Drawing for the job (mm, zero at the part's lowest x, y, z). A direction names the side the tool comes from. Coordinates: 2 decimals unless noted, no trailing zeros. Order: outer loops, then holes, each group sorted by start corner. A loop starts at its lowest first (then second) coordinate and runs counter-clockwise, first axis right, second up. Notation, with made-up numbers: (-15, 14.25) - (-5, 14.25) arc R20 ccw to (-5, 52.25) - close; hole circle Ø3 at (68, 19). An arc over 180 degrees is marked (long way). Answer as CSV lines item,"result". Start each with the question number.
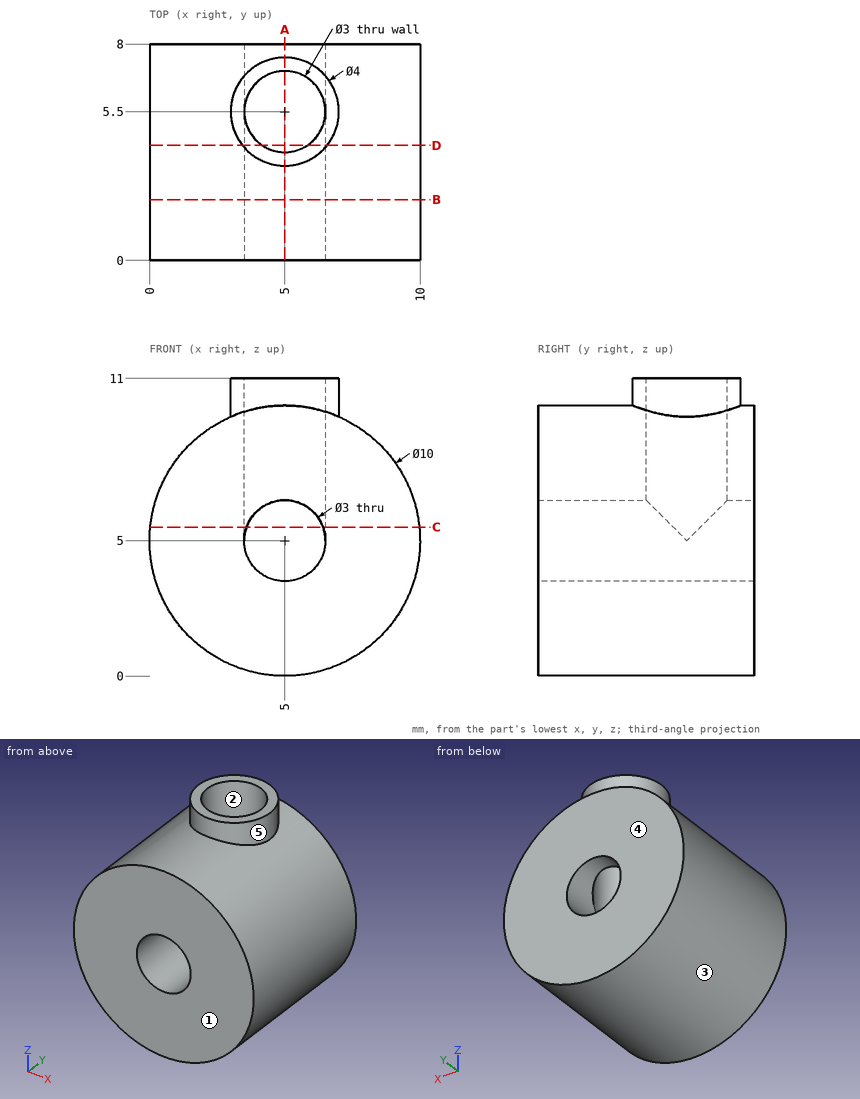
(1) Band-saw the part on D-D on y = 4.25. List the corners of the cut face in (x, z), plus the area to 3 significant figures.
(2) Drop a flat-ended pin along its axis: pin 1 Ø3 at (y, z) = (3.5, 3) entering from -X. Give the stop position or say it passes through.
(3) Probe L1, parallel to X at y = 2, z = 5; L2, parallel to Z at x = 3.75, y = 3; L3, parallel to Y at x = 5.5, z = 7.5. List the from-to ranges inside material, lowest first. Write a range as [from, to].
(4) Band-saw the part on B-B on y = 2.25. List the corners of the cut face in (x, z).
(5) Band-saw the part on A-A on x = 5. List the corners of the cut face in (y, z), plus the area to 3 significant figures.
(6) Pull direction X, two halves, no side cores. Call the marked faces 1, 2 and 3: +X half, -X half, draft (parallel to the pull), parting line (faces both ways), or undercut.
(7) Band-saw the part on C-C on z = 5.5. List the corners of the cut face in (x, y), plus the area to 3 significant figures.
(8) Which spindle directions (+Z, -Z, +X, -X, +Y, -Y) get a long thin tool onto all of the face, cutting with end or side? Do the marked faces 4 and 5. Say none if no direction does.
Filled in:
1,outline,"(3.44, 9.75) arc R5 ccw (long way) to (6.56, 9.75) - (6.56, 11) - (5.83, 11) - (5.83, 6.25) arc R1.5 cw (long way) to (4.17, 6.25) - (4.17, 11) - (3.44, 11) - close"
1,area,"67.3 mm^2"
2,pin 1,"stops at x = 0.03"
3,L1,"x = [0, 3.5], [6.5, 10]"
3,L2,"z = [0.16, 4.17], [5.83, 9.84]"
3,L3,"y = [0, 4.09], [6.91, 8]"
4,outline,"circle Ø10 at (5, 5); hole circle Ø3 at (5, 5)"
5,outline,"(0, 0) - (8, 0) - (8, 3.5) - (0, 3.5) - close; (0, 6.5) - (4, 6.5) - (4, 11) - (3.5, 11) - (3.5, 10) - (0, 10) - close; (7, 6.5) - (8, 6.5) - (8, 10) - (7.5, 10) - (7.5, 11) - (7, 11) - close"
5,area,"46.5 mm^2"
6,face 1,"draft"
6,face 2,"undercut"
6,face 3,"parting line"
7,outline,"(0.03, 0) - (3.59, 0) - (3.59, 5) arc R1.5 cw to (3.59, 6) - (3.59, 8) - (0.03, 8) - close; (6.41, 0) - (9.97, 0) - (9.97, 8) - (6.41, 8) - (6.41, 6) arc R1.5 cw to (6.41, 5) - close"
7,area,"56.9 mm^2"
8,face 4,"+Z, -Z, +X, -X, +Y"
8,face 5,"+Z"
